Check sheet for the modelled part. Datum: model origin and axes. Units: mm. Face numbers are marked on the shaded views. Coordinates: 2 decimals unless noted, no trailing zeros. Write each loop counter-clockwise with the first axis right and the second up, starting at its lowest first coordinate (ties: lowest second). Pieces come first, ordered by that corner, then holes. Notation, with made-up numbers: (83.5, 21) -> (117.5, 21) arc R15 ccw to (117.5, 43) -> close; hole circle Ø2 at (-9, -29.75). An arc over 180 degrees is marked (long way). One line per item, written item: value. Start each with the question number.
1) Draft check along Y on the marked faces 1, 2 and 3. Enter one of: +Y half, -Y half, draft (parallel to the pull), parting line (faces both ways), or undercut.
2) Gauge pin test, flat ends, axial feed: P1, Ø2, axis at y = 7.5, z = 2.5, coming from the +X side; P2, Ø2.5, axis at x = 0, y = 16, coming from the -Z side; P3, Ø1, axis at x = 6, z = 0.5, coming from the +Y side; P4, Ø1.5, axis at y = -14, z = 1.5, coming from the -X side. Record the tip position at first contact, or that the pin passes through.
3) Sectioned sample at A-A on y = 0. Enter the section's corners in (x, z), plus the area to 3 significant figures.
4) Sectioned sample at C-C on x = -16. Enter the section's corners in (y, z), plus the area to 3 significant figures.
5) Sectioned sample at D-D on z = 1.65. Enter the section's corners in (x, y).
6) Sectioned sample at B-B on x = 0.5. Enter the section's corners in (y, z).
7) Scan lines: line 1 along Y through (x, z) = (0, 4); line 2 along Y through (x, z) = (0, 4.55); line 3 along X through (y, z) = (-1, 0.45). Record each from-to range of solid material in increasing order. Write a range as [from, to].
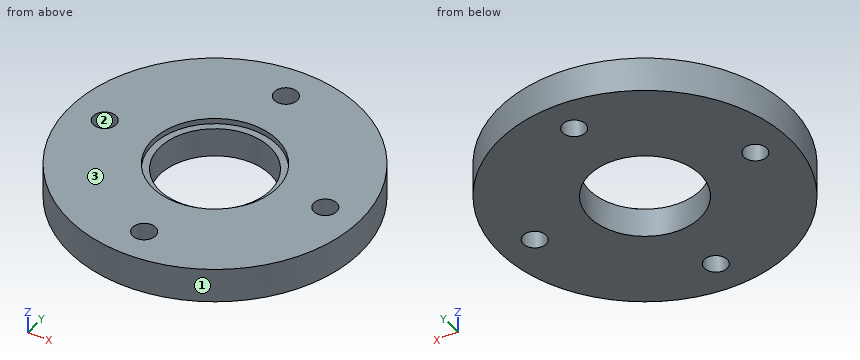
```python
from build123d import *

# Parameters (mm, degrees)
SKETCH_1_R          = 21
SKETCH_1_R_2        = 8
EXTRUDE_1_DEPTH     = 5
M4X0_71_D           = 3.3
SKETCH_4_R          = 9
CUT_EXTRUDE_1_DEPTH = 0.8


with BuildPart() as part:
    # Эскиз1 → Бобышка-Вытянуть1 (new body)
    with BuildSketch(Plane.XY):
        Circle(SKETCH_1_R)
        Circle(SKETCH_1_R_2, mode=Mode.SUBTRACT)
    extrude(amount=EXTRUDE_1_DEPTH)

    # Отверстие обработанное метчиком M4x0.71 (through all)
    with Locations(Plane.XY.offset(5)):
        with Locations((0, 16), (-16, 0), (0, -16), (16, 0)):
            Hole(M4X0_71_D / 2)

    # Эскиз4 → Вырез-Вытянуть1 (cut)
    with BuildSketch(Plane.XY.offset(5)):
        Circle(SKETCH_4_R)
    extrude(amount=-CUT_EXTRUDE_1_DEPTH, mode=Mode.SUBTRACT)


solid = part.part
```
Answers:
1. face 1: parting line
1. face 2: undercut
1. face 3: draft
2. P1: stops at x = 19.97
2. P2: passes through
2. P3: stops at y = 20.27
2. P4: stops at x = -16.29
3. outline: (-21, 0) -> (-17.65, 0) -> (-17.65, 5) -> (-21, 5) -> close; (-14.35, 0) -> (-8, 0) -> (-8, 4.2) -> (-9, 4.2) -> (-9, 5) -> (-14.35, 5) -> close; (8, 0) -> (14.35, 0) -> (14.35, 5) -> (9, 5) -> (9, 4.2) -> (8, 4.2) -> close; (17.65, 0) -> (21, 0) -> (21, 5) -> (17.65, 5) -> close
3. area: 95.4 mm2
4. outline: (-13.6, 0) -> (-1.65, 0) -> (-1.65, 5) -> (-13.6, 5) -> close; (1.65, 0) -> (13.6, 0) -> (13.6, 5) -> (1.65, 5) -> close
4. area: 120 mm2
5. outline: circle Ø42 at (0, 0); hole circle Ø3.3 at (-16, 0); hole circle Ø16 at (0, 0); hole circle Ø3.3 at (0, -16); hole circle Ø3.3 at (0, 16); hole circle Ø3.3 at (16, 0)
6. outline: (-20.99, 0) -> (-17.57, 0) -> (-17.57, 5) -> (-20.99, 5) -> close; (-14.43, 0) -> (-7.98, 0) -> (-7.98, 4.2) -> (-8.99, 4.2) -> (-8.99, 5) -> (-14.43, 5) -> close; (7.98, 0) -> (14.43, 0) -> (14.43, 5) -> (8.99, 5) -> (8.99, 4.2) -> (7.98, 4.2) -> close; (17.57, 0) -> (20.99, 0) -> (20.99, 5) -> (17.57, 5) -> close
7. line 1: y = [-21, -17.65], [-14.35, -8], [8, 14.35], [17.65, 21]
7. line 2: y = [-21, -17.65], [-14.35, -9], [9, 14.35], [17.65, 21]
7. line 3: x = [-20.98, -17.31], [-14.69, -7.94], [7.94, 14.69], [17.31, 20.98]
